```python
from build123d import *

# Parameters (mm, degrees)
F0_R     = 10.668
F0_R_2   = 1.5875
F0_R_3   = 2.54
F1_DEPTH = 11.684


with BuildPart() as f1:
    # F0 (on Front) → F1 (new body)
    with BuildSketch(Plane.XZ):
        with BuildLine():
            ThreePointArc((-23.759524406, 15.875), (0, 28.575), (23.759524406, 15.875))
            Line((23.759524406, 15.875), (28.575, 15.875))
            Line((28.575, 15.875), (28.575, 147.0559814834))
            ThreePointArc((28.575, 147.0559814834), (30.0665512939, 151.1447436641), (33.8405043055, 153.312687413))
            Line((33.8405043055, 153.312687413), (70.9344956945, 159.742312587))
            ThreePointArc((70.9344956945, 159.742312587), (74.7084487061, 161.9102563359), (76.2, 165.9990185166))
            Line((76.2, 165.9990185166), (76.2, 203.2))
            Line((76.2, 203.2), (17.526, 203.2))
            Line((17.526, 203.2), (-17.526, 203.2))
            Line((-17.526, 203.2), (-76.2, 203.2))
            Line((-76.2, 203.2), (-76.2, 165.9990185166))
            ThreePointArc((-76.2, 165.9990185166), (-74.7084487061, 161.9102563359), (-70.9344956945, 159.742312587))
            Line((-70.9344956945, 159.742312587), (-33.8405043055, 153.312687413))
            ThreePointArc((-33.8405043055, 153.312687413), (-30.0665512939, 151.1447436641), (-28.575, 147.0559814834))
            Line((-28.575, 147.0559814834), (-28.575, 15.875))
            Line((-28.575, 15.875), (-23.759524406, 15.875))
        make_face()
        with Locations((-50.8, 184.15)):
            Circle(F0_R, mode=Mode.SUBTRACT)
        with Locations((-25.4, 184.15)):
            Circle(F0_R_2, mode=Mode.SUBTRACT)
        with Locations((25.4, 184.15)):
            Circle(F0_R_2, mode=Mode.SUBTRACT)
        with Locations((50.8, 184.15)):
            Circle(F0_R, mode=Mode.SUBTRACT)
        with BuildLine():
            Line((-60.325, -15.875), (-23.759524406, -15.875))
            ThreePointArc((-23.759524406, -15.875), (-27.3446433045, -8.2946433045), (-28.575, 0))
            Line((-28.575, 0), (-28.575, 15.875))
            Line((-28.575, 15.875), (-60.325, 15.875))
            ThreePointArc((-60.325, 15.875), (-62.5700640303, 14.9450640303), (-63.5, 12.7))
            Line((-63.5, 12.7), (-63.5, -12.7))
            ThreePointArc((-63.5, -12.7), (-62.5700640303, -14.9450640303), (-60.325, -15.875))
        make_face()
        with Locations((-50.8, 0)):
            Circle(F0_R_3, mode=Mode.SUBTRACT)
        with BuildLine():
            ThreePointArc((28.575, 0), (27.3446433045, -8.2946433045), (23.759524406, -15.875))
            Line((23.759524406, -15.875), (60.325, -15.875))
            ThreePointArc((60.325, -15.875), (62.5700640303, -14.9450640303), (63.5, -12.7))
            Line((63.5, -12.7), (63.5, 12.7))
            ThreePointArc((63.5, 12.7), (62.5700640303, 14.9450640303), (60.325, 15.875))
            Line((60.325, 15.875), (28.575, 15.875))
            Line((28.575, 15.875), (28.575, 0))
        make_face()
        with Locations((50.8, 0)):
            Circle(F0_R_3, mode=Mode.SUBTRACT)
        with BuildLine():
            Line((23.759524406, -15.875), (7.4259713843, -15.875))
            ThreePointArc((7.4259713843, -15.875), (0, -17.526), (-7.4259713843, -15.875))
            Line((-7.4259713843, -15.875), (-23.759524406, -15.875))
            ThreePointArc((-23.759524406, -15.875), (0, -28.575), (23.759524406, -15.875))
        make_face()
        with BuildLine():
            ThreePointArc((-7.4259713843, -15.875), (-17.526, 0), (-7.4259713843, 15.875))
            Line((-7.4259713843, 15.875), (-23.759524406, 15.875))
            ThreePointArc((-23.759524406, 15.875), (-27.3446433045, 8.2946433045), (-28.575, 0))
            ThreePointArc((-28.575, 0), (-27.3446433045, -8.2946433045), (-23.759524406, -15.875))
            Line((-23.759524406, -15.875), (-7.4259713843, -15.875))
        make_face()
        with BuildLine():
            ThreePointArc((-7.4259713843, 15.875), (0, 17.526), (7.4259713843, 15.875))
            Line((7.4259713843, 15.875), (23.759524406, 15.875))
            ThreePointArc((23.759524406, 15.875), (0, 28.575), (-23.759524406, 15.875))
            Line((-23.759524406, 15.875), (-7.4259713843, 15.875))
        make_face()
        with BuildLine():
            ThreePointArc((7.4259713843, 15.875), (14.7869579441, 9.4077920236), (17.526, 0))
            ThreePointArc((17.526, 0), (14.7869579441, -9.4077920236), (7.4259713843, -15.875))
            Line((7.4259713843, -15.875), (23.759524406, -15.875))
            ThreePointArc((23.759524406, -15.875), (27.3446433045, -8.2946433045), (28.575, 0))
            ThreePointArc((28.575, 0), (27.3446433045, 8.2946433045), (23.759524406, 15.875))
            Line((23.759524406, 15.875), (7.4259713843, 15.875))
        make_face()
        with BuildLine():
            ThreePointArc((-28.575, 0), (-27.3446433045, 8.2946433045), (-23.759524406, 15.875))
            Line((-23.759524406, 15.875), (-28.575, 15.875))
            Line((-28.575, 15.875), (-28.575, 0))
        make_face()
        with BuildLine():
            Line((28.575, 15.875), (23.759524406, 15.875))
            ThreePointArc((23.759524406, 15.875), (27.3446433045, 8.2946433045), (28.575, 0))
            Line((28.575, 0), (28.575, 15.875))
        make_face()
    extrude(amount=F1_DEPTH)


solid = f1.part
```
Part model, mm, in its own coordinate system. A direction names the side the tool comes from. Round coordinates to 2 decimals unless told otherwise and drop trailing zeros. Loops run counter-clockwise (first coordinate to the right, second up) from the corner with the lowest first, then second, coordinate; pieces in that order, holes last. Notation, with made-up numbers: (55.5, -18) -> (70.5, -18) arc R19 cw to (70.5, -4) -> close; hole circle Ø9 at (33, 5.25). An arc over 180 degrees is marked (long way). Use CSV: the item, a comma, the result in double quotes. Start each with the question number.
1) Cut at A-A, the plane y = -2.25. Give the number of separate pieces and of enclosed holes in the cut face, plus the area to 3 significant figures.
2) Cut at B-B, the plane x = 50.8. Write the cut outline in (y, z) (3 decimals).
3) Drop flat-ended pins along their axis: P1, Ø6, axis at x = -41.5, y = -7, coming from the -Z side (3 decimals); P2, Ø6, axis at y = -8, z = 6, coming from the +X side; P3, Ø6, axis at y = -6, z = 15.5, coming from the -X side; P4, Ø17, axis at x = 50.8, z = 184.15, coming from the +Y side. Give the stop position or say it passes through.
4) Cut at C-C, the plane z = 100. Write the cut outline in (x, y) (3 decimals), plus the area to 3 significant figures.
5) Cut at D-D, the plane x = -66. Write the cut outline in (y, z), plus the area to 3 significant figures.
6) Pull direction X, two halves, no side cores. Call faces 5 (the cylindrical face through (55.723, -5.76, 174.686)), 6 (the cylindrical face through (-30.107, -5.76, 151.192)), 7 (the flat face through (45, -6, 15.875)), 8 (the cylindrical face through (53.223, -5.76, 0.763)): +X half, -X half, draft (parallel to the pull), parting line (faces both ways), or undercut.
7) Wall check: L1, parallel to Z at x = -50.8, y = -8.5 (3 decimals); L2, parallel to X at y = -2.5, z = 192.5; L3, parallel to Z at x = 25.4, y = -7.5 (1 decimal). Give the ranges that are in metal, low to high. Write a range as [from, to].
8) Which spindle directions (+Z, -Z, +X, -X, +Y, -Y) get a long thin tool onto all of the face, cutting with end or side? Do faces 1 (the flat face through (-28.575, -6, 82)), 2 (the flat face through (63.5, -6, 0)), 3 (the flat face through (-63.5, -6, 0)), 4 (the cylindrical face through (30.03, -5.76, 151.1)). Say none if no direction does.
Determined:
1,separate pieces,"1"
1,enclosed holes,"7"
1,area,"17,900 mm2"
2,outline,"(-11.684, -15.875) -> (0, -15.875) -> (0, -2.54) -> (-11.684, -2.54) -> close; (-11.684, 2.54) -> (0, 2.54) -> (0, 15.875) -> (-11.684, 15.875) -> close; (-11.684, 156.252) -> (0, 156.252) -> (0, 173.482) -> (-11.684, 173.482) -> close; (-11.684, 194.818) -> (0, 194.818) -> (0, 203.2) -> (-11.684, 203.2) -> close"
3,P1,"stops at z = -15.875"
3,P2,"stops at x = 63.5"
3,P3,"stops at x = -63.5"
3,P4,"passes through"
4,outline,"(-28.575, -11.684) -> (28.575, -11.684) -> (28.575, 0) -> (-28.575, 0) -> close"
4,area,"668 mm2"
5,outline,"(-11.68, 158.89) -> (0, 158.89) -> (0, 203.2) -> (-11.68, 203.2) -> close"
5,area,"518 mm2"
6,face 5,"undercut"
6,face 6,"-X half"
6,face 7,"draft"
6,face 8,"undercut"
7,L1,"z = [-15.875, -2.54], [2.54, 15.875], [156.252, 173.482], [194.818, 203.2]"
7,L2,"x = [-76.2, -57.44], [-44.16, 44.16], [57.44, 76.2]"
7,L3,"z = [-15.9, 182.6], [185.7, 203.2]"
8,face 1,"-X, +Y, -Y"
8,face 2,"-Z, +X, +Y, -Y"
8,face 3,"-Z, -X, +Y, -Y"
8,face 4,"+X, +Y, -Y"
